Could you check a few things on this model? Use its own coordinates, in mm. Round coordinates to 2 decimals unless told otherwise and drop trailing zeros. Loops run counter-clockwise (first coordinate to the right, second up) from the corner with the lowest first, then second, coordinate; pieces in that order, holes last. Notation, with made-up numbers: (32.25, 76) - (37.25, 76) arc R21 cw to (37.25, 95) - close; hole circle Ø6 at (45, 10). An arc over 180 degrees is marked (long way). Use one line per item in the form item = value.
```python
from build123d import *
from build123d.topology import SkipClean

# Parameters (mm, degrees)
SKETCH_1_R      = 2.75
EXTRUDE_1_DEPTH = 49
EXTRUDE_START   = 7
EXTRUDE_2_DEPTH = 7
EXTRUDE_START_2 = -12
SKETCH_6_R      = 11
SKETCH_6_W      = 1.25
SKETCH_6_H      = 3.5
SKETCH_6_W_2    = 3.5
SKETCH_6_H_2    = 1.25
EXTRUDE_4_DEPTH = 2
EXTRUDE_START_3 = -27.9
SKETCH_7_R      = 5
EXTRUDE_5_DEPTH = 2.5


with BuildPart() as part:
    # Sketch 1 → Extrude 1 (new body)
    with BuildSketch(Plane(origin=(0, 0, 0), x_dir=(1, 0, 0), z_dir=(0, 1, 0))):
        with Locations(Location((0, 0, 0), (0, 0, 270))):
            Circle(SKETCH_1_R)
    extrude(amount=EXTRUDE_1_DEPTH)

    # Sketch 2 → Extrude 2 (add)
    with SkipClean():  # the faces are left unmerged after this step: merging them gives an invalid solid
        with BuildSketch(Plane.XZ.offset(EXTRUDE_START)):
            with BuildLine():
                Line((-1.95, 1.939071943), (-1.95, -1.939071943))
                ThreePointArc((-1.95, -1.939071943), (0, -2.75), (1.95, -1.939071943))
                Line((1.95, -1.939071943), (1.95, 1.939071943))
                ThreePointArc((1.95, 1.939071943), (0, 2.75), (-1.95, 1.939071943))
            make_face()
        extrude(amount=-EXTRUDE_2_DEPTH)

    # Sketch 6 → Extrude 4 (add)
    with SkipClean():  # the faces are left unmerged after this step: merging them gives an invalid solid
        with BuildSketch(Plane(origin=(0, 49, 0), x_dir=(1, 0, 0), z_dir=(0, 1, 0)).offset(EXTRUDE_START_2)):
            with Locations(Location((0, 0, 0), (0, 0, 270))):
                Circle(SKETCH_6_R)
            Polygon((2.495759621, 9.703700784), (3.684580266, 9.317429541), (2.603020786, 5.988731734), (1.414200141, 6.375002977), align=None, mode=Mode.SUBTRACT)
            with Locations((0, 8.25)):
                Rectangle(SKETCH_6_W, SKETCH_6_H, mode=Mode.SUBTRACT)
            Polygon((5.372216901, 8.457535726), (6.383488144, 7.722804161), (4.326239761, 4.891244681), (3.314968518, 5.625976246), align=None, mode=Mode.SUBTRACT)
            Polygon((7.722804161, 6.383488144), (8.457535726, 5.372216901), (5.625976246, 3.314968518), (4.891244681, 4.326239761), align=None, mode=Mode.SUBTRACT)
            Polygon((9.317429541, 3.684580266), (9.703700784, 2.495759621), (6.375002977, 1.414200141), (5.988731734, 2.603020786), align=None, mode=Mode.SUBTRACT)
            with Locations((8.25, 0)):
                Rectangle(SKETCH_6_W_2, SKETCH_6_H_2, mode=Mode.SUBTRACT)
            Polygon((9.703700784, -2.495759621), (9.317429541, -3.684580266), (5.988731734, -2.603020786), (6.375002977, -1.414200141), align=None, mode=Mode.SUBTRACT)
            Polygon((8.457535726, -5.372216901), (7.722804161, -6.383488144), (4.891244681, -4.326239761), (5.625976246, -3.314968518), align=None, mode=Mode.SUBTRACT)
            Polygon((6.383488144, -7.722804161), (5.372216901, -8.457535726), (3.314968518, -5.625976246), (4.326239761, -4.891244681), align=None, mode=Mode.SUBTRACT)
            Polygon((3.684580266, -9.317429541), (2.495759621, -9.703700784), (1.414200141, -6.375002977), (2.603020786, -5.988731734), align=None, mode=Mode.SUBTRACT)
            with Locations((0, -8.25)):
                Rectangle(SKETCH_6_W, SKETCH_6_H, mode=Mode.SUBTRACT)
            Polygon((-2.495759621, -9.703700784), (-3.684580266, -9.317429541), (-2.603020786, -5.988731734), (-1.414200141, -6.375002977), align=None, mode=Mode.SUBTRACT)
            Polygon((-5.372216901, -8.457535726), (-6.383488144, -7.722804161), (-4.326239761, -4.891244681), (-3.314968518, -5.625976246), align=None, mode=Mode.SUBTRACT)
            Polygon((-7.722804161, -6.383488144), (-8.457535726, -5.372216901), (-5.625976246, -3.314968518), (-4.891244681, -4.326239761), align=None, mode=Mode.SUBTRACT)
            Polygon((-9.317429541, -3.684580266), (-9.703700784, -2.495759621), (-6.375002977, -1.414200141), (-5.988731734, -2.603020786), align=None, mode=Mode.SUBTRACT)
            with Locations((-8.25, 0)):
                Rectangle(SKETCH_6_W_2, SKETCH_6_H_2, mode=Mode.SUBTRACT)
            Polygon((-9.703700784, 2.495759621), (-9.317429541, 3.684580266), (-5.988731734, 2.603020786), (-6.375002977, 1.414200141), align=None, mode=Mode.SUBTRACT)
            Polygon((-8.457535726, 5.372216901), (-7.722804161, 6.383488144), (-4.891244681, 4.326239761), (-5.625976246, 3.314968518), align=None, mode=Mode.SUBTRACT)
            Polygon((-6.383488144, 7.722804161), (-5.372216901, 8.457535726), (-3.314968518, 5.625976246), (-4.326239761, 4.891244681), align=None, mode=Mode.SUBTRACT)
            Polygon((-3.684580266, 9.317429541), (-2.495759621, 9.703700784), (-1.414200141, 6.375002977), (-2.603020786, 5.988731734), align=None, mode=Mode.SUBTRACT)
        extrude(amount=EXTRUDE_4_DEPTH)

    # Sketch 7 → Extrude 5 (add)
    with SkipClean():  # the faces are left unmerged after this step: merging them gives an invalid solid
        with BuildSketch(Plane(origin=(0, 49, 0), x_dir=(1, 0, 0), z_dir=(0, 1, 0)).offset(EXTRUDE_START_3)):
            with Locations(Location((0, 0, 0), (0, 0, 270))):
                Circle(SKETCH_7_R)
        extrude(amount=-EXTRUDE_5_DEPTH)


solid = part.part
```
1. For P1, Ø1, axis at y = 37.5, z = -8, coming from the +X side; P2, Ø1, axis at y = 38, z = 8.5, coming from the -X side; P3, Ø1.2, axis at y = -3.5, z = 0, coming from the -X side, each with a flat end and sliding along its axis, tell me the tip position at first contact or that it passes through.
Solution:
P1 = 8.05
P2 = -7.55
P3 = -1.95
2. If we section it at B-B, the plane y = 33.5: Write out the boundary of the cut face in (x, z), plus the area to 3 significant figures.
Solution:
outline = circle Ø5.5 at (0, 0)
area = 23.8 mm^2
3. We'd pull the mould along X, two halves only. Please class faces 1 (the face through (-10.74, 37.99, -2.38)), 2 (the face through (1.95, -4, 0)), 3 (the face through (-3.082, 37.986, 9.513)): +X half, -X half, draft (parallel to the pull), parting line (faces both ways), or undercut.
Solution:
face_1 = parting line
face_2 = +X half
face_3 = undercut
4. Please list where these lines run through material, in increasing order: line 1 along Y through (x, z) = (-3, 2); line 2 along Y through (x, z) = (-4.25, 4.75); line 3 along Z through (x, y) = (0, 42).
Solution:
line_1 = 18.6 to 21.1, 37 to 39
line_2 = 37 to 39
line_3 = -2.75 to 2.75
5. If we section it at A-A, the plane z = 0: Count the separate pieces of the cut face and the enclosed holes in it, plus the area to 3 significant figures.
Solution:
separate_pieces = 3
enclosed_holes = 0
area = 327 mm^2
